Read the model definition and answer for the solid it produces. Units are mm, in the model's axes. A direction names the side the tool comes from. Round coordinates to 2 decimals unless told otherwise and drop trailing zeros. Write each loop counter-clockwise with the first axis right and the second up, starting at its lowest first coordinate (ties: lowest second). Pieces come first, ordered by that corner, then holes. Notation, with made-up numbers: (-13, 57.25) -> (29, 57.25) arc R32 ccw to (29, 89.25) -> close; hole circle Ø2 at (1, 53.25). An arc over 180 degrees is marked (long way). Return JSON: item names as keys, results as strings. Group by question number.
(1) The mould has two halves that part along Z. Classify faces 6 (the flat face through (21, 3.5, 68)), 7 (the flat face through (12, 7, 54)), 8 (the cylindrical face through (-22.43, 12.46, 5.65)), 9 (the flat face through (0, 13, -10.5)): released by +Z, released by -Z, zero draft, split by the parting line, or undercut.
(2) Given pin 1 (8 mm diameter, centred on y = 1.5, z = 47.5, fed in from -X); pin 2 (18 mm diameter, centred on x = 18.5, z = 64.5, fed in from -Y); pin 3 (2 mm diameter, centred on y = 10.5, z = 56, fed in from +X), each flat-ended and moving along its own axis, determine where each tip first touches the part or whether it passes through.
(3) A cutting plane is placed at C-C on y = 13.75. Give the vertices of the cut face in (x, z), then the cut area to 3 significant figures.
(4) A cutting plane is placed at B-B on z = 5. Give the vertices of the cut face in (x, y), then the cut area to 3 significant figures.
(5) A cutting plane is placed at A-A on x = 7.5. Give the vertices of the cut face in (y, z), then the cut area to 3 significant figures.
(6) For faces 1 (the flat face through (21, 12.5, 38)), 2 (the flat face through (0, 5, -20)), 3 (the flat face through (0, 5, 17)), 4 (the flat face through (-12, 7, 24)), 5 (the cylindrical face through (14.81, 7.412, 36.002)), determine the directions among +Z, -Z, +X, -X, +Y, -Y from which every point of the face is accessible in a straight line to the end or side of a thin tool.
(7) Straight lines are drawn through the part: line 1 (X direction, y = 12.25, z = -7.5); line 2 (Z direction, x = 16.25, y = 7.5); line 3 (Z direction, x = -19, y = 9.25) (3 decimals). For each, find the intervals that lie inside material, in ascending order.
```python
from build123d import *
from OCP.BRepFilletAPI import BRepFilletAPI_MakeChamfer

# Parameters (mm, degrees)
BODY_DEPTH                = 15
TONG_THINNING_CUT_DEPTH   = 95.731198662
LOWER_CUTOUT_DEPTH        = 109.853112036
SKETCH10_W                = 41
SKETCH10_H                = 21
SERVO_CUTOUT_DEPTH        = 91.410176418
SKETCH12_R                = 2
ROPE_TUNNEL_ROUNDS_R      = 0.5
TONG_CHAMFERS_SIZE        = 2
TONG_CHAMFERS_SIZE2       = 2.200726077
LARGER_CHAMFERS_SIZE      = 5
TONG_TIP_THINNER_DEPTH    = 95.73119871
TONG_TIP_HOLE_D           = 3.4
TONG_TIP_HOLE_CSINK_D     = 3.7
TONG_TIP_HOLE_CSINK_ANGLE = 90
GUIDING_RAIL_DEPTH        = 45
MOUTNING_FLATTENER_DEPTH  = 109.853112101


# Read off the part's stored shape, not the designer's step: guiding_screw_holes, servo_connector_holes, mouting_holes
with BuildPart() as part:
    # Sketch2 → body (new body)
    with BuildSketch(Plane(origin=(0, 0, 0), x_dir=(1, 0, 0), z_dir=(0, 1, 0))):
        Polygon((-35, 25), (35, 25), (35, -22), (32, -25), (27, -82), (13, -82), (13, -55), (10, -52), (10, -22), (-35, -22), align=None)
    extrude(amount=BODY_DEPTH)

    # Sketch3 → tong_thinning_cut (cut, through all)
    with BuildSketch(Plane.ZY.offset(-10)):
        Polygon((22, 15), (82, 15), (82, 12.5), (24.5, 12.5), align=None)
        Polygon((82, 0), (22, 0), (24.5, 2.5), (82, 2.5), align=None)
    extrude(amount=-TONG_THINNING_CUT_DEPTH, mode=Mode.SUBTRACT)

    # guiding_screw_holes outline → guiding_screw_holes (revolve, cut)
    with BuildSketch(Plane(origin=(0, 7.5, 46), x_dir=(0, 1, 0), z_dir=(0, 0, -1))):
        Polygon((1.85, 20), (0, 21.111592145), (0, 10), (2.15, 10), (1.85, 10.3), align=None)
    revolve(axis=Axis((0, 7.5, 46), (1, 0, 0)), mode=Mode.SUBTRACT)

    # guiding_screw_holes 2 outline → guiding_screw_holes 2 (revolve, cut)
    with BuildSketch(Plane(origin=(0, 7.5, 30), x_dir=(0, 1, 0), z_dir=(0, 0, -1))):
        Polygon((1.85, 20), (0, 21.111592145), (0, 10), (2.15, 10), (1.85, 10.3), align=None)
    revolve(axis=Axis((0, 7.5, 30), (1, 0, 0)), mode=Mode.SUBTRACT)

    # Sketch9 → lower_cutout (cut, through all)
    with BuildSketch(Plane(origin=(35, 0, 0), x_dir=(0, 0, -1), z_dir=(1, 0, 0))):
        Polygon((-19.5, 0), (-14.5, 10), (12, 10), (17, 0), align=None)
    extrude(amount=-LOWER_CUTOUT_DEPTH, mode=Mode.SUBTRACT)

    # Sketch10 → servo_cutout (cut, through all)
    with BuildSketch(Plane(origin=(0, 15, 0), x_dir=(1, 0, 0), z_dir=(0, 1, 0))):
        Rectangle(SKETCH10_W, SKETCH10_H)
    extrude(amount=-SERVO_CUTOUT_DEPTH, mode=Mode.SUBTRACT)

    # rope_tunnel_cutout: sweep along a path in Sketch11
    with BuildLine(Plane(origin=(0, 7.5, 0), x_dir=(1, 0, 0), z_dir=(0, 1, 0))) as rope_tunnel_cutout_path:
        Line((10, -38), (19, -38))
        ThreePointArc((19, -38), (24.656854249, -35.656854249), (27, -30))
        Line((27, -30), (27, -10))
    # Sketch12 → rope_tunnel_cutout (sweep, cut)
    with BuildSketch(Plane.ZY.offset(-10)):
        with Locations((38, 7.5)):
            Circle(SKETCH12_R)
    sweep(path=rope_tunnel_cutout_path.line, mode=Mode.SUBTRACT)

    # rope_tunnel_rounds
    rope_tunnel_rounds_edges = [part.edges().sort_by_distance(p)[0] for p in [
        (10, 7.5, 36),
        (25, 7.499978341, 15.750010829),
    ]]
    fillet(rope_tunnel_rounds_edges, radius=ROPE_TUNNEL_ROUNDS_R)

    # tong_chamfers: one chamfer whose edges measure the first distance from different faces: ONE call of the kernel's chamfer builder (chamfer() names one face for all edges)
    tong_chamfers_edges_1 = [part.edges().sort_by_distance(p)[0] for p in [
        (27, 7.5, 82),
    ]]
    tong_chamfers_side_1 = [part.faces().sort_by_distance(p)[0] for p in [
        (20, 7.5, 82),
    ]]
    tong_chamfers_edges_2 = [part.edges().sort_by_distance(p)[0] for p in [
        (13, 7.5, 82),
    ]]
    tong_chamfers = BRepFilletAPI_MakeChamfer(part.part.solid().wrapped)
    for e in tong_chamfers_edges_1:
        tong_chamfers.Add(TONG_CHAMFERS_SIZE, TONG_CHAMFERS_SIZE2, e.wrapped, tong_chamfers_side_1[0].wrapped)  # the first distance lies on this face
    for e in tong_chamfers_edges_2:
        tong_chamfers.Add(TONG_CHAMFERS_SIZE, e.wrapped)
    add(Compound.cast(tong_chamfers.Shape()), mode=Mode.REPLACE)

    # servo_connector_holes outline → servo_connector_holes (revolve, cut)
    with BuildSketch(Plane(origin=(24, 0, 5), x_dir=(1, 0, 0), z_dir=(0, 0, 1))):
        Polygon((0, 10), (1.7, 10), (1.7, 14.85), (1.85, 15), (0, 15), align=None)
    revolve(axis=Axis((24, 0, 5), (0, 1, 0)), mode=Mode.SUBTRACT)

    # servo_connector_holes 2 outline → servo_connector_holes 2 (revolve, cut)
    with BuildSketch(Plane(origin=(24, 0, -5), x_dir=(1, 0, 0), z_dir=(0, 0, 1))):
        Polygon((0, 10), (1.7, 10), (1.7, 14.85), (1.85, 15), (0, 15), align=None)
    revolve(axis=Axis((24, 0, -5), (0, 1, 0)), mode=Mode.SUBTRACT)

    # servo_connector_holes 3 outline → servo_connector_holes 3 (revolve, cut)
    with BuildSketch(Plane(origin=(-24, 0, 5), x_dir=(1, 0, 0), z_dir=(0, 0, 1))):
        Polygon((0, 10), (1.7, 10), (1.7, 14.85), (1.85, 15), (0, 15), align=None)
    revolve(axis=Axis((-24, 0, 5), (0, 1, 0)), mode=Mode.SUBTRACT)

    # servo_connector_holes 4 outline → servo_connector_holes 4 (revolve, cut)
    with BuildSketch(Plane(origin=(-24, 0, -5), x_dir=(1, 0, 0), z_dir=(0, 0, 1))):
        Polygon((0, 10), (1.7, 10), (1.7, 14.85), (1.85, 15), (0, 15), align=None)
    revolve(axis=Axis((-24, 0, -5), (0, 1, 0)), mode=Mode.SUBTRACT)

    # larger_chamfers
    larger_chamfers_edges = [part.edges().sort_by_distance(p)[0] for p in [
        (-35, 7.5, -25),
        (35, 7.5, -25),
    ]]
    chamfer(larger_chamfers_edges, length=LARGER_CHAMFERS_SIZE)

    # Sketch16 → tong_tip_thinner (cut, through all)
    with BuildSketch(Plane.ZY.offset(-10)):
        Polygon((52, 12.5), (55, 11.5), (82, 11.5), (82, 12.5), align=None)
        Polygon((52, 2.5), (55, 3.5), (82, 3.5), (82, 2.5), align=None)
    extrude(amount=-TONG_TIP_THINNER_DEPTH, mode=Mode.SUBTRACT)

    # tong_tip_hole (through all)
    with Locations(Plane(origin=(0, 11.5, 0), x_dir=(1, 0, 0), z_dir=(0, 1, 0))):
        with Locations((19, -74)):
            CounterSinkHole(TONG_TIP_HOLE_D / 2, TONG_TIP_HOLE_CSINK_D / 2, counter_sink_angle=TONG_TIP_HOLE_CSINK_ANGLE)

    # Sketch18 → guiding_rail (add)
    with BuildSketch(Plane.ZY.offset(-10)):
        Polygon((22, 10), (22, 5), (24, 6), (24, 9), align=None)
    extrude(amount=GUIDING_RAIL_DEPTH)

    # Sketch19 → moutning_flattener (cut, through all)
    with BuildSketch(Plane.ZY.offset(35)):
        Polygon((-14.5, 5), (-25, 5), (-25, 0), (-17, 0), align=None)
    extrude(amount=-MOUTNING_FLATTENER_DEPTH, mode=Mode.SUBTRACT)

    # mouting_holes outline → mouting_holes (revolve, cut)
    with BuildSketch(Plane(origin=(20, 0, -20), x_dir=(1, 0, 0), z_dir=(0, 0, 1))):
        Polygon((0, 5), (2.25, 5), (2.25, 14.975), (2.275, 15), (0, 15), align=None)
    revolve(axis=Axis((20, 0, -20), (0, 1, 0)), mode=Mode.SUBTRACT)

    # mouting_holes 2 outline → mouting_holes 2 (revolve, cut)
    with BuildSketch(Plane(origin=(-20, 0, -20), x_dir=(1, 0, 0), z_dir=(0, 0, 1))):
        Polygon((0, 5), (2.25, 5), (2.25, 14.975), (2.275, 15), (0, 15), align=None)
    revolve(axis=Axis((-20, 0, -20), (0, 1, 0)), mode=Mode.SUBTRACT)


solid = part.part
```
Checks:
{
 "1": {"face 6": "zero draft", "face 7": "released by +Z", "face 8": "undercut", "face 9": "undercut"},
 "2": {"pin 1": "stops at x = 10", "pin 2": "stops at y = 3.5", "pin 3": "stops at x = 29.37"},
 "3": {"outline": "(-35, -20) -> (-30, -25) -> (30, -25) -> (35, -20) -> (35, 22) -> (33.75, 23.25) -> (10, 23.25) -> (10, 22) -> (-35, 22) -> close; hole circle Ø3.4 at (-24, -5); hole circle Ø3.4 at (-24, 5); hole circle Ø4.5 at (-20, -20); hole (-20.5, -10.5) -> (20.5, -10.5) -> (20.5, 10.5) -> (-20.5, 10.5) -> close; hole circle Ø4.5 at (20, -20); hole circle Ø3.4 at (24, -5); hole circle Ø3.4 at (24, 5)", "area": "2,370 mm^2"},
 "4": {"outline": "(-35, 10) -> (-25.7, 10) -> (-25.7, 14.85) -> (-25.85, 15) -> (-35, 15) -> close; (-22.3, 10) -> (-20.5, 10) -> (-20.5, 15) -> (-22.15, 15) -> (-22.3, 14.85) -> close; (20.5, 10) -> (22.3, 10) -> (22.3, 14.85) -> (22.15, 15) -> (20.5, 15) -> close; (25.7, 10) -> (35, 10) -> (35, 15) -> (25.85, 15) -> (25.7, 14.85) -> close", "area": "111 mm^2"},
 "5": {"outline": "(0, 19.5) -> (10, 14.5) -> (10, 10.5) -> (15, 10.5) -> (15, 22) -> (10, 22) -> (9, 24) -> (6, 24) -> (5, 22) -> (0, 22) -> close; (5, -25) -> (15, -25) -> (15, -10.5) -> (10, -10.5) -> (10, -12) -> (5, -14.5) -> close", "area": "247 mm^2"},
 "6": {"face 1": "+Z, +X, -X, +Y", "face 2": "-Z, +X, -X, -Y", "face 3": "+X, -X, -Y", "face 4": "+Z, -X, +Y, -Y", "face 5": "-X"},
 "7": {"line 1": "x = -35 to -20.5, 20.5 to 35", "line 2": "z = -25 to -13.25, 15.75 to 28.15, 31.85 to 36, 40 to 44.15, 47.85 to 82", "line 3": "z = -25 to -22.016, -17.984 to -12.375, 14.875 to 23.5"}
}
